Geometry check sheet. Reference: the model listing, model coordinates, mm. Coordinates: 2 decimals unless noted, no trailing zeros. Write each loop counter-clockwise with the first axis right and the second up, starting at its lowest first coordinate (ties: lowest second). Pieces come first, ordered by that corner, then holes. Notation, with made-up numbers: (58.5, 0) -> (68.5, 0) arc R25 ccw to (68.5, 38) -> close; hole circle Ø8 at (-23, 80). An arc over 180 degrees is marked (long way). Use a Markdown table: item, result.
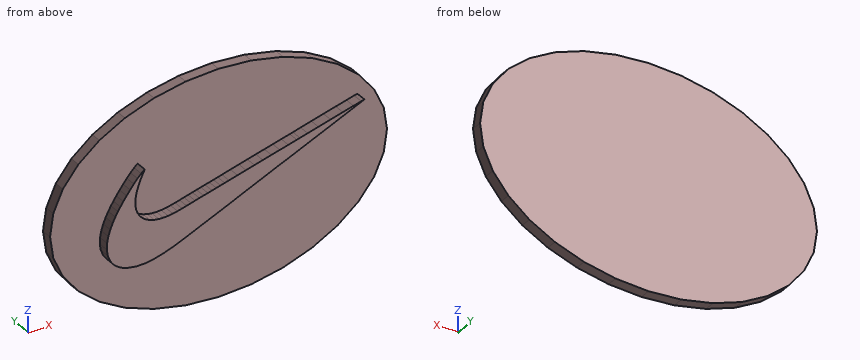
```python
from build123d import *

# Parameters (mm, degrees)
F1_DEPTH = 3.175
F2_DEPTH = 6.35


# Not quite as in the source:
# - a length typed as a fraction of an inch, garbled in the dataset ("3 / 203.2 mm" for 3/8 in), is restored


with BuildPart() as f1:
    # F0 (on Front) → F1 (new body)
    with BuildSketch(Plane.XZ):
        Polygon((46.7098888, -6.1941202), (47.625, 0), (46.7098888, 6.1941202), (43.9997596, 12.150217), (39.598727, 17.6393602), (33.675955, 22.4506536), (26.4590276, 26.3991598), (18.2252874, 29.33319), (9.2911676, 31.1399428), (0, 31.75), (-9.291193, 31.1399428), (-18.2253128, 29.33319), (-26.459053, 26.3991598), (-33.6759804, 22.4506536), (-39.5987524, 17.6393602), (-43.999785, 12.150217), (-46.7099142, 6.1941202), (-47.625, 0), (-46.7099142, -6.1941202), (-43.999785, -12.1501916), (-39.5987524, -17.6393602), (-33.6759804, -22.4506282), (-26.459053, -26.3991598), (-18.2253128, -29.3331646), (-9.291193, -31.1399174), (0, -31.75), (9.2911676, -31.1399174), (18.2252874, -29.3331646), (26.4590276, -26.3991598), (33.675955, -22.4506282), (39.598727, -17.6393602), (43.9997596, -12.1501916), align=None)
        Polygon((38.341681, 12.2114056), (39.2552936, 12.4328174), (27.5334984, 7.2016112), (26.0539992, 6.5582038), (24.5790974, 5.9062112), (23.1074976, 5.2491132), (21.6381838, 4.590415), (20.1697844, 3.9334948), (18.7011818, 3.2820102), (17.2311822, 2.6391108), (15.7585918, 2.008505), (15.0165816, 1.6895064), (14.2783814, 1.3633196), (13.5421878, 1.0321036), (12.8065784, 0.6979158), (12.0698768, 0.362712), (11.3305844, 0.028702), (10.5870756, -0.3020822), (9.8377756, -0.6275832), (3.9710868, -3.244596), (2.5708864, -3.8890956), (1.1199876, -4.5439838), (-0.366014, -5.2049934), (-1.8718022, -5.8679842), (-3.38201, -6.5287906), (-4.8813212, -7.1831962), (-6.3541148, -7.8269846), (-7.7852016, -8.4560918), (-9.9900232, -9.4423992), (-12.3777248, -10.4928924), (-14.8971, -11.5218972), (-17.497425, -12.4434854), (-20.1276204, -13.1720844), (-22.7367084, -13.6216898), (-25.2738128, -13.706602), (-27.6880066, -13.341096), (-28.5486094, -13.0792982), (-29.3320216, -12.7701802), (-30.0423072, -12.4116846), (-30.6835048, -12.0018048), (-31.2595006, -11.5384834), (-31.774511, -11.0196884), (-32.2323206, -10.4433878), (-32.6370188, -9.8076004), (-33.312608, -8.1586832), (-33.575625, -6.422898), (-33.4963008, -4.6470824), (-33.1451204, -2.8779978), (-32.5923148, -1.1624818), (-31.9084198, 0.4526026), (-31.1636156, 1.9203162), (-30.4284126, 3.1938976), (-29.7318176, 4.2935144), (-28.9025076, 5.5216044), (-27.9718008, 6.8250054), (-26.9710154, 8.1507076), (-25.9315204, 9.4455996), (-24.8846086, 10.6565192), (-23.8617252, 11.7305074), (-22.8942138, 12.614402), (-22.9568248, 12.4025152), (-23.0575104, 12.1500138), (-23.185501, 11.8695978), (-23.3301032, 11.5739164), (-23.6254036, 10.9873034), (-23.857204, 10.491597), (-24.207724, 9.6268032), (-24.5462044, 8.744204), (-24.8575068, 7.8445106), (-25.1264166, 6.9283072), (-25.3376176, 5.9964066), (-25.4759206, 5.0494946), (-25.5260094, 4.0882062), (-25.4729234, 3.1132018), (-25.225121, 1.8998184), (-24.779605, 0.8263128), (-24.1524028, -0.1045972), (-23.3597196, -0.8900922), (-22.417405, -1.5274036), (-21.3416134, -2.0136866), (-20.1485246, -2.3462996), (-18.8540136, -2.5223978), (-17.5612044, -2.5464008), (-16.2439096, -2.449195), (-14.9162008, -2.2540976), (-13.591921, -1.9846036), (-12.2850148, -1.6639032), (-11.009503, -1.3152882), (-9.7794064, -0.9621012), (-8.6086188, -0.6277864), (-7.4149204, -0.2975864), (-6.2186058, 0.028702), (-5.0205132, 0.3525012), (-3.8219126, 0.6751066), (-2.6237184, 0.9980168), (-1.4270228, 1.3224002), (-0.2328164, 1.6497046), (0.9576816, 1.9814032), (3.358388, 2.652903), (5.7565798, 3.3170114), (8.152892, 3.9752016), (10.547985, 4.6289976), (12.942697, 5.2796186), (15.3375868, 5.928614), (17.7332894, 6.5773046), (20.1306938, 7.227316), (21.0277964, 7.4752962), (23.2002838, 8.0761078), (26.2238998, 8.910701), (29.6740834, 9.860407), (33.1267816, 10.806303), (36.1573826, 11.6296186), align=None, mode=Mode.SUBTRACT)
    extrude(amount=F1_DEPTH)

    # F0 (on Front) → F2 (join)
    with BuildSketch(Plane.XZ):
        Polygon((27.5334984, 7.2016112), (39.2552936, 12.4328174), (38.341681, 12.2114056), (36.1573826, 11.6296186), (33.1267816, 10.806303), (29.6740834, 9.860407), (26.2238998, 8.910701), (23.2002838, 8.0761078), (21.0277964, 7.4752962), (20.1306938, 7.227316), (17.7332894, 6.5773046), (15.3375868, 5.928614), (12.942697, 5.2796186), (10.547985, 4.6289976), (8.152892, 3.9752016), (5.7565798, 3.3170114), (3.358388, 2.652903), (0.9576816, 1.9814032), (-0.2328164, 1.6497046), (-1.4270228, 1.3224002), (-2.6237184, 0.9980168), (-3.8219126, 0.6751066), (-5.0205132, 0.3525012), (-6.2186058, 0.028702), (-7.4149204, -0.2975864), (-8.6086188, -0.6277864), (-9.7794064, -0.9621012), (-11.009503, -1.3152882), (-12.2850148, -1.6639032), (-13.591921, -1.9846036), (-14.9162008, -2.2540976), (-16.2439096, -2.449195), (-17.5612044, -2.5464008), (-18.8540136, -2.5223978), (-20.1485246, -2.3462996), (-21.3416134, -2.0136866), (-22.417405, -1.5274036), (-23.3597196, -0.8900922), (-24.1524028, -0.1045972), (-24.779605, 0.8263128), (-25.225121, 1.8998184), (-25.4729234, 3.1132018), (-25.5260094, 4.0882062), (-25.4759206, 5.0494946), (-25.3376176, 5.9964066), (-25.1264166, 6.9283072), (-24.8575068, 7.8445106), (-24.5462044, 8.744204), (-24.207724, 9.6268032), (-23.857204, 10.491597), (-23.6254036, 10.9873034), (-23.3301032, 11.5739164), (-23.185501, 11.8695978), (-23.0575104, 12.1500138), (-22.9568248, 12.4025152), (-22.8942138, 12.614402), (-23.8617252, 11.7305074), (-24.8846086, 10.6565192), (-25.9315204, 9.4455996), (-26.9710154, 8.1507076), (-27.9718008, 6.8250054), (-28.9025076, 5.5216044), (-29.7318176, 4.2935144), (-30.4284126, 3.1938976), (-31.1636156, 1.9203162), (-31.9084198, 0.4526026), (-32.5923148, -1.1624818), (-33.1451204, -2.8779978), (-33.4963008, -4.6470824), (-33.575625, -6.422898), (-33.312608, -8.1586832), (-32.6370188, -9.8076004), (-32.2323206, -10.4433878), (-31.774511, -11.0196884), (-31.2595006, -11.5384834), (-30.6835048, -12.0018048), (-30.0423072, -12.4116846), (-29.3320216, -12.7701802), (-28.5486094, -13.0792982), (-27.6880066, -13.341096), (-25.2738128, -13.706602), (-22.7367084, -13.6216898), (-20.1276204, -13.1720844), (-17.497425, -12.4434854), (-14.8971, -11.5218972), (-12.3777248, -10.4928924), (-9.9900232, -9.4423992), (-7.7852016, -8.4560918), (-6.3541148, -7.8269846), (-4.8813212, -7.1831962), (-3.38201, -6.5287906), (-1.8718022, -5.8679842), (-0.366014, -5.2049934), (1.1199876, -4.5439838), (2.5708864, -3.8890956), (3.9710868, -3.244596), (9.8377756, -0.6275832), (10.5870756, -0.3020822), (11.3305844, 0.028702), (12.0698768, 0.362712), (12.8065784, 0.6979158), (13.5421878, 1.0321036), (14.2783814, 1.3633196), (15.0165816, 1.6895064), (15.7585918, 2.008505), (17.2311822, 2.6391108), (18.7011818, 3.2820102), (20.1697844, 3.9334948), (21.6381838, 4.590415), (23.1074976, 5.2491132), (24.5790974, 5.9062112), (26.0539992, 6.5582038), align=None)
    extrude(amount=F2_DEPTH)


solid = f1.part
```
Item 1: Section check C-C on z = 25. Record the boundary of the cut face in (x, y) (3 decimals).
Answer block:
| item | result |
|---|---|
| outline | (-29.016, -3.175) -> (29.016, -3.175) -> (29.016, 0) -> (-29.016, 0) -> close |
Item 2: Thickness scan on L1, parallel to Y at x = -40, z = -0.5 (3 decimals); L2, parallel to Z at x = -3.5, y = -5.25; L3, parallel to Z at x = 39, y = -1. Record the ranges inside material, lowest first. Write a range as [from, to].
Answer block:
| item | result |
|---|---|
| L1 | y = [-3.175, 0] |
| L2 | z = [-6.58, 0.76] |
| L3 | z = [-18.13, 18.13] |
Item 3: Depth check by flat-ended pin: P1, Ø1, axis at x = 11, z = 15.5, coming from the +Y side; P2, Ø10, axis at x = -38, z = 15.5, coming from the -Y side (3 decimals). Enter the tip coordinate at first touch or a pass-through.
Answer block:
| item | result |
|---|---|
| P1 | stops at y = 0 |
| P2 | stops at y = -3.175 |
Item 4: Section check B-B on z = -20. Record the boundary of the cut face in (x, y) (3 decimals).
Answer block:
| item | result |
|---|---|
| outline | (-36.693, -3.175) -> (36.693, -3.175) -> (36.693, 0) -> (-36.693, 0) -> close |
